from build123d import *

# Parameters (mm, degrees)
SKETCH1_R             = 1.55
BOSS_EXTRUDE1_DEPTH   = 60
BOSS_EXTRUDE1_2_DEPTH = 60
BOSS_EXTRUDE1_3_DEPTH = 60
BOSS_EXTRUDE1_4_DEPTH = 60
BOSS_EXTRUDE2_DEPTH   = 40
SHELL1_T              = -3


with BuildPart() as part:
    # Sketch1 → Boss-Extrude1 (new body)
    with BuildSketch(Plane(origin=(0, 0, 0), x_dir=(1, 0, 0), z_dir=(0, 1, 0))):
        with Locations(Location((-76.5, 52.45, 0), (0, 0, 270))):
            Circle(SKETCH1_R)
    extrude(amount=BOSS_EXTRUDE1_DEPTH)



with BuildPart() as body_2:
    # Sketch1 → Boss-Extrude1 2 (new body)
    with BuildSketch(Plane(origin=(0, 0, 0), x_dir=(1, 0, 0), z_dir=(0, 1, 0))):
        with Locations(Location((76.5, 52.45, 0), (0, 0, 270))):
            Circle(SKETCH1_R)
    extrude(amount=BOSS_EXTRUDE1_2_DEPTH)


with BuildPart() as body_3:
    # Sketch1 → Boss-Extrude1 3 (new body)
    with BuildSketch(Plane(origin=(0, 0, 0), x_dir=(1, 0, 0), z_dir=(0, 1, 0))):
        with Locations(Location((76.5, -52.45, 0), (0, 0, 270))):
            Circle(SKETCH1_R)
    extrude(amount=BOSS_EXTRUDE1_3_DEPTH)


with BuildPart() as body_4:
    # Sketch1 → Boss-Extrude1 4 (new body)
    with BuildSketch(Plane(origin=(0, 0, 0), x_dir=(1, 0, 0), z_dir=(0, 1, 0))):
        with Locations(Location((-76.5, -52.45, 0), (0, 0, 270))):
            Circle(SKETCH1_R)
    extrude(amount=BOSS_EXTRUDE1_4_DEPTH)


with BuildPart() as part_1:
    add(part.part)

    add(body_2.part)  # Boss-Extrude2 merges body 2

    add(body_3.part)  # Boss-Extrude2 merges body 3

    add(body_4.part)  # Boss-Extrude2 merges body 4
    # Sketch2 → Boss-Extrude2 (add)
    with BuildSketch(Plane(origin=(0, 0, 0), x_dir=(1, 0, 0), z_dir=(0, 1, 0))):
        with BuildLine():
            Line((-78.05, 52.45), (-78.05, -52.45))
            ThreePointArc((-78.05, -52.45), (-77.596015511, -53.546015511), (-76.5, -54))
            Line((-76.5, -54), (76.5, -54))
            ThreePointArc((76.5, -54), (77.596015511, -53.546015511), (78.05, -52.45))
            Line((78.05, -52.45), (78.05, 52.45))
            ThreePointArc((78.05, 52.45), (77.596015511, 53.546015511), (76.5, 54))
            Line((76.5, 54), (-76.5, 54))
            ThreePointArc((-76.5, 54), (-77.596015511, 53.546015511), (-78.05, 52.45))
        make_face()
    extrude(amount=BOSS_EXTRUDE2_DEPTH)

    # Shell1
    shell1_openings = [part_1.faces().sort_by_distance(p)[0] for p in [
        (0, 40, 0),
    ]]
    offset(amount=SHELL1_T, openings=shell1_openings)


solid = part_1.part
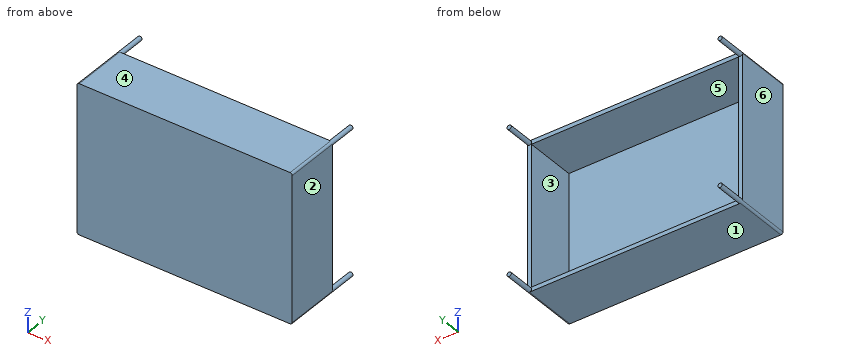
Read the model definition and answer for the solid it produces. Units are mm, in the model's axes. Face numbers are marked on the shaded views. A direction names the side the tool comes from. Give positions to 0.01 mm unless a question says otherwise; leave off trailing zeros. Write each loop counter-clockwise with the first axis right and the second up, starting at its lowest first coordinate (ties: lowest second). Pieces come first, ordered by that corner, then holes. Notation, with made-up numbers: (-13.75, 74.25) -> (15.25, 74.25) arc R9 cw to (15.25, 89.25) -> close; hole circle Ø5 at (71.5, 68.25). An arc over 180 degrees is marked (long way). Answer as a JSON object with one key per item and string values. Group by question number.
1) Consider L1, parallel to Z at x = 0, y = 24; L2, parallel to X at y = 35.5, z = 39.5; L3, parallel to Y at x = -7, z = 18. Determine where each line is inside the solid, lowest interval first. Write a range as from..to.
2) Find section A-A (y = 33). Write down the section's boundary in (x, z), and give its area (3 significant figures).
3) The mould has two halves that part along Z. Classify the marked faces 1, 2, 3 and 4: +Z half, -Z half, draft (parallel to the pull), parting line (faces both ways), or undercut.
4) Find section C-C (z = 41). Write down the section's boundary in (x, y).
5) A tool of negligible diameter and unlimited length cuts with its end or side. For the marked faces 5 and 6, from which of +Z, -Z, +X, -X, +Y, -Y can it reach the whole face along a straight path? Write none if from no direction.
6) This flat-tipped pin is pushed along its axis until it touches: P1, Ø8, axis at x = -46.5, z = -9, coming from the +Y side. Where does it stop, or does it pass through?
7) Find section B-B (x = -42). Write down the section's boundary in (y, z).
8) Find section D-D (y = 45.5). Write down the section's boundary in (x, z), and give its area (3 significant figures).
Values follow:
{
 "1": {"L1": "z = -54..-51, 51..54", "L2": "x = -78.05..-75.05, 75.05..78.05", "L3": "y = 0..3"},
 "2": {"outline": "(-78.05, -52.45) arc R1.55 ccw to (-76.5, -54) -> (76.5, -54) arc R1.55 ccw to (78.05, -52.45) -> (78.05, 52.45) arc R1.55 ccw to (76.5, 54) -> (-76.5, 54) arc R1.55 ccw to (-78.05, 52.45) -> close; hole (-75.05, -51) -> (75.05, -51) -> (75.05, 51) -> (-75.05, 51) -> close", "area": "1,550 mm2"},
 "3": {"face 1": "-Z half", "face 2": "draft", "face 3": "undercut", "face 4": "+Z half"},
 "4": {"outline": "(-78.05, 0) -> (78.05, 0) -> (78.05, 40) -> (75.05, 40) -> (75.05, 3) -> (-75.05, 3) -> (-75.05, 40) -> (-78.05, 40) -> close"},
 "5": {"face 5": "+Y", "face 6": "+Z, -Z, -X, +Y, -Y"},
 "6": {"P1": "stops at y = 3"},
 "7": {"outline": "(0, -54) -> (40, -54) -> (40, -51) -> (3, -51) -> (3, 51) -> (40, 51) -> (40, 54) -> (0, 54) -> close"},
 "8": {"outline": "circle Ø3.1 at (-76.5, -52.45); circle Ø3.1 at (-76.5, 52.45); circle Ø3.1 at (76.5, -52.45); circle Ø3.1 at (76.5, 52.45)", "area": "30.2 mm2"}
}
